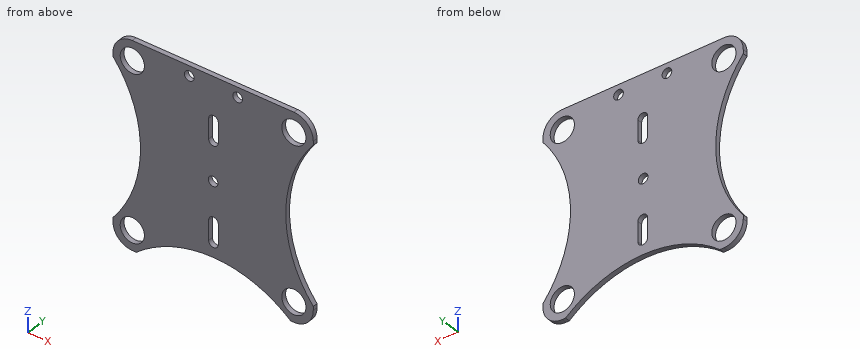
from build123d import *

# Parameters (mm, degrees)
SKETCH1_R           = 5
SKETCH1_R_2         = 2
BOSS_EXTRUDE1_DEPTH = 2


with BuildPart() as part:
    # Sketch1 → Boss-Extrude1 (new body)
    with BuildSketch(Plane(origin=(0, 0, 0), x_dir=(1, 0, 0), z_dir=(0, 1, 0))):
        with BuildLine():
            Line((32.038903515, 41.368938053), (33.368938053, 41.368938053))
            ThreePointArc((33.368938053, 41.368938053), (39.025792302, 39.025792302), (41.368938053, 33.368938053))
            Line((41.368938053, 33.368938053), (41.368938053, 31.743362343))
            ThreePointArc((41.368938053, 31.743362343), (30, 0), (41.368938053, -31.743362343))
            Line((41.368938053, -31.743362343), (41.368938053, -33.368938053))
            ThreePointArc((41.368938053, -33.368938053), (39.025792302, -39.025792302), (33.368938053, -41.368938053))
            Line((33.368938053, -41.368938053), (32.038903515, -41.368938053))
            Line((32.038903515, -41.368938053), (-31.743362343, -41.368938053))
            Line((-31.743362343, -41.368938053), (-33.368938053, -41.368938053))
            ThreePointArc((-33.368938053, -41.368938053), (-39.025792302, -39.025792302), (-41.368938053, -33.368938053))
            Line((-41.368938053, -33.368938053), (-41.368938053, -31.743362343))
            ThreePointArc((-41.368938053, -31.743362343), (-30, 0), (-41.368938053, 31.743362343))
            Line((-41.368938053, 31.743362343), (-41.368938053, 33.368938053))
            ThreePointArc((-41.368938053, 33.368938053), (-39.025792302, 39.025792302), (-33.368938053, 41.368938053))
            Line((-33.368938053, 41.368938053), (-31.743362343, 41.368938053))
            ThreePointArc((-31.743362343, 41.368938053), (0.147770586, 29.90602396), (32.038903515, 41.368938053))
        make_face()
        with Locations((-33.368938053, 33.368938053)):
            Circle(SKETCH1_R, mode=Mode.SUBTRACT)
        with Locations((33.368938053, 33.368938053)):
            Circle(SKETCH1_R, mode=Mode.SUBTRACT)
        with Locations((-33.368938053, -33.368938053)):
            Circle(SKETCH1_R, mode=Mode.SUBTRACT)
        with Locations((33.368938053, -33.368938053)):
            Circle(SKETCH1_R, mode=Mode.SUBTRACT)
        Circle(SKETCH1_R_2, mode=Mode.SUBTRACT)
        with Locations((10.147770586, -37.36127525)):
            Circle(SKETCH1_R_2, mode=Mode.SUBTRACT)
        with Locations((-9.852229414, -37.36127525)):
            Circle(SKETCH1_R_2, mode=Mode.SUBTRACT)
        with BuildLine():
            Line((2.147770586, 24), (2.147770586, 16))
            ThreePointArc((2.147770586, 16), (0.147770586, 14), (-1.852229414, 16))
            Line((-1.852229414, 16), (-1.852229414, 24))
            ThreePointArc((-1.852229414, 24), (0.147770586, 26), (2.147770586, 24))
        make_face(mode=Mode.SUBTRACT)
        with BuildLine():
            Line((-1.852229414, -24), (-1.852229414, -16))
            ThreePointArc((-1.852229414, -16), (0.147770586, -14), (2.147770586, -16))
            Line((2.147770586, -16), (2.147770586, -24))
            ThreePointArc((2.147770586, -24), (0.147770586, -26), (-1.852229414, -24))
        make_face(mode=Mode.SUBTRACT)
    extrude(amount=BOSS_EXTRUDE1_DEPTH)


solid = part.part
Part model, mm, in its own coordinate system. Round coordinates to 2 decimals unless told otherwise and drop trailing zeros. Write each loop counter-clockwise with the first axis right and the second up, starting at its lowest first coordinate (ties: lowest second). Pieces come first, ordered by that corner, then holes. Notation, with made-up numbers: M 68,45 L 97,45 A4 ccw 97,51 Z; hole C 59.5,23.25 d11. An arc over 180 degrees is marked long. Return JSON: item names as keys, results as strings. Group by question number.
(1) Saw through at B-B on y = 0.55. Count the separate pieces of the cut face and the enclosed holes in it, then the cut area to 3 significant figures.
(2) Pin check, flat tips, straight feed: pin 1 Ø4.5 at (x, z) = (0, 0) entering from +Y; pin 2 Ø0.6 at (y, z) = (1.5, -18) entering from +X; pin 3 Ø1 at (y, z) = (1, 20.5) entering from -X. Stop position of each tip, or through.
(3) Saw through at D-D on z = 17.5. Write the cut outline in (x, y), then the cut area to 3 significant figures.
(4) Saw through at C-C on x = 0. Write the cut outline in (y, z).
(5) Saw through at A-A on z = 0. Write the cut outline in (x, y).
(6) Drill centre lines: probe 1 along X at (y, z) = (1.6, 32); probe 2 along X at (y, z) = (0.3, 37); probe 3 along X at (y, z) = (1, 36.5). Where is each one in solid material? Low to high.
Returned:
{
 "1": {"separate pieces": "1", "enclosed holes": "9", "area": "4,860 mm²"},
 "2": {"pin 1": "y = 2", "pin 2": "x = 33.47", "pin 3": "x = -34.62"},
 "3": {"outline": "M -33.16,0 L -1.85,0 L -1.85,2 L -33.16,2 Z; M 2.15,0 L 33.16,0 L 33.16,2 L 2.15,2 Z", "area": "125 mm²"},
 "4": {"outline": "M 0,-29.91 L 2,-29.91 L 2,-25.99 L 0,-25.99 Z; M 0,-14.01 L 2,-14.01 L 2,-2 L 0,-2 Z; M 0,2 L 2,2 L 2,14.01 L 0,14.01 Z; M 0,25.99 L 2,25.99 L 2,41.37 L 0,41.37 Z"},
 "5": {"outline": "M -30,0 L -2,0 L -2,2 L -30,2 Z; M 2,0 L 30,0 L 30,2 L 2,2 Z"},
 "6": {"probe 1": "-41.37 to -38.18, -28.56 to 28.56, 38.18 to 41.37", "probe 2": "-40.5 to -36.81, -29.93 to -11.82, -7.89 to 8.18, 12.11 to 29.93, 36.81 to 40.5", "probe 3": "-40.73 to -37.27, -29.47 to -11.66, -8.05 to 8.34, 11.95 to 29.47, 37.27 to 40.73"}
}
